Check sheet for the modelled part. Datum: model origin and axes. Units: mm. Round coordinates to 2 decimals unless told otherwise and drop trailing zeros. Loops run counter-clockwise (first coordinate to the right, second up) from the corner with the lowest first, then second, coordinate; pieces in that order, holes last. Notation, with made-up numbers: (51, 62) - (103, 62) arc R31 ccw to (103, 89) - close; hole circle Ø1 at (45.25, 12.5). An arc over 180 degrees is marked (long way). Put each result on its own line as item: value.
Autodesk Inventor part; units mm, degrees
ref_plane "YZ Plane" through (0, 0, 0) normal (1, 0, 0) x (0, 1, 0)
ref_plane "XZ Plane" through (0, 0, 0) normal (0, 1, 0) x (-1, 0, 0)
ref_plane "XY Plane" through (0, 0, 0) normal (0, 0, 1) x (1, 0, 0)
sketch "Sketch1" plane through (0, 0, 0) normal (1, 0, 0) x (0, 1, 0)
  line L0 (0, 0) -> (-50, 0)
  line L1 (-50, 0) -> (-50, -20)
  line L2 (-50, -20) -> (0, -20)
  line L3 (0, -20) -> (0, 0)
  line L4 (0, 0) -> (0, -10)
  line L5 (0, -10) -> (-10, -10)
  line L6 (-10, -10) -> (-23, -10)
  line L7 (-23, -10) -> (-40, -10)
  line L8 (-40, -10) -> (-45, -10)
  circle A0 centre (-10, -10) radius 1.5
  circle A1 centre (-23, -10) radius 1.5
  circle A2 centre (-40, -10) radius 1.5
  circle A3 centre (-45, -10) radius 1.5
  dimension "d0" = 50
  dimension "d1" = 20
  dimension "d2" = 10
  dimension "d3" = 10
  dimension "d4" = 13
  dimension "d5" = 17
  dimension "d7" = 5
  dimension "d8" = 3
  dimension "d9" = 3
  dimension "d10" = 3
  dimension "d11" = 3
extrude "Extrusion1" add sketch "Sketch1" along normal blind 1.5
sketch "Sketch2" plane through (0, 0, 0) normal (-1, 0, 0) x (0, 0, 1)
  line L0 (-20, 0) -> (0, 0)
  line L1 (0, 0) -> (-20, 0)
  line L2 (-20, 0) -> (-20, 10)
  line L3 (-20, 10) -> (0, 10)
  line L4 (0, 10) -> (0, 0)
  circle A0 centre (-10, -10) radius 1.5
  line L5 (-10, -10) -> (-10, 5)
  line L6 (-10, 5) -> (-5, 5)
  line L7 (-5, 5) -> (-15, 5)
  circle A1 centre (-5, 5) radius 1.5
  circle A2 centre (-15, 5) radius 1.5
  dimension "d14" = 10
  dimension "d15" = 20
  dimension "d16" = 15
  dimension "d17" = 5
  dimension "d18" = 10
  dimension "d19" = 3
  dimension "d20" = 3
extrude "Extrusion2" add sketch "Sketch2" against normal blind 1.5 contours L2 L3 L4 L0
sketch "Sketch3" plane through (1.5, 0, 0) normal (1, 0, 0) x (0, 0, -1)
  circle A0 centre (10, -10) radius 1.5
  circle A1 centre (10, -10) radius 1.5
  point P0 (0, 0)
extrude "Extrusion3" add sketch "Sketch3" against normal blind 1.5
sketch "Sketch5" plane through (0, 0, 0) normal (-1, 0, 0) x (0, 0, 1)
  line L0 (0, 10) -> (0, -50)
  line L1 (0, 10) -> (0, -3.388)
  line L2 (0, -3.388) -> (-6.5, -3.388)
  circle A0 centre (-6.5, -3.388) radius 2
  point P0 (0, 0)
  dimension "d30" = 13.388
  dimension "d31" = 6.5
  dimension "d32" = 4
extrude "Extrusion5" cut sketch "Sketch5" against normal blind 1.5
properties part number "plateLocker"
Item 1: Thickness scan on line 1 (Z direction, x = 0.35, y = -23); line 2 (Y direction, x = 1.45, z = -6.25); line 3 (Y direction, x = 0.65, z = -6). Record the ranges inside material, lowest first. Write a range as from..to.
Filled sheet:
line 1: -20..-11.5, -8.5..0
line 2: -50..-5.37, -1.4..4.17, 5.83..10
line 3: -50..-5.32, -1.45..3.88, 6.12..10
Item 2: Section check A-A on z = -10. Enter the section's corners in (x, y).
Filled sheet:
outline: (0, -50) - (1.5, -50) - (1.5, -46.5) - (0, -46.5) - close; (0, -43.5) - (1.5, -43.5) - (1.5, -41.5) - (0, -41.5) - close; (0, -38.5) - (1.5, -38.5) - (1.5, -24.5) - (0, -24.5) - close; (0, -21.5) - (1.5, -21.5) - (1.5, 10) - (0, 10) - close
Item 3: Section check C-C on y = 5. Enter the section's corners in (x, z).
Filled sheet:
outline: (0, -20) - (1.5, -20) - (1.5, -16.5) - (0, -16.5) - close; (0, -13.5) - (1.5, -13.5) - (1.5, -6.5) - (0, -6.5) - close; (0, -3.5) - (1.5, -3.5) - (1.5, 0) - (0, 0) - close
Item 4: Section check B-B on y = -23. Enter the section's corners in (x, z), then the cut area to 3 significant figures.
Filled sheet:
outline: (0, -20) - (1.5, -20) - (1.5, -11.5) - (0, -11.5) - close; (0, -8.5) - (1.5, -8.5) - (1.5, 0) - (0, 0) - close
area: 25.5 mm²
Item 5: Section check D-D on z = -5.75. Enter the section's corners in (x, y).
Filled sheet:
outline: (0, -50) - (1.5, -50) - (1.5, -5.24) - (0, -5.24) - close; (0, -1.53) - (1.5, -1.53) - (1.5, 3.7) - (0, 3.7) - close; (0, 6.3) - (1.5, 6.3) - (1.5, 10) - (0, 10) - close
Item 6: Go/stop test with a flat-tipped pin: pin 1 (2.5 mm diameter, centred on y = -23, z = -10, fed in from -X). Record where the tip stops, or that it passes through.
Filled sheet:
pin 1: through
